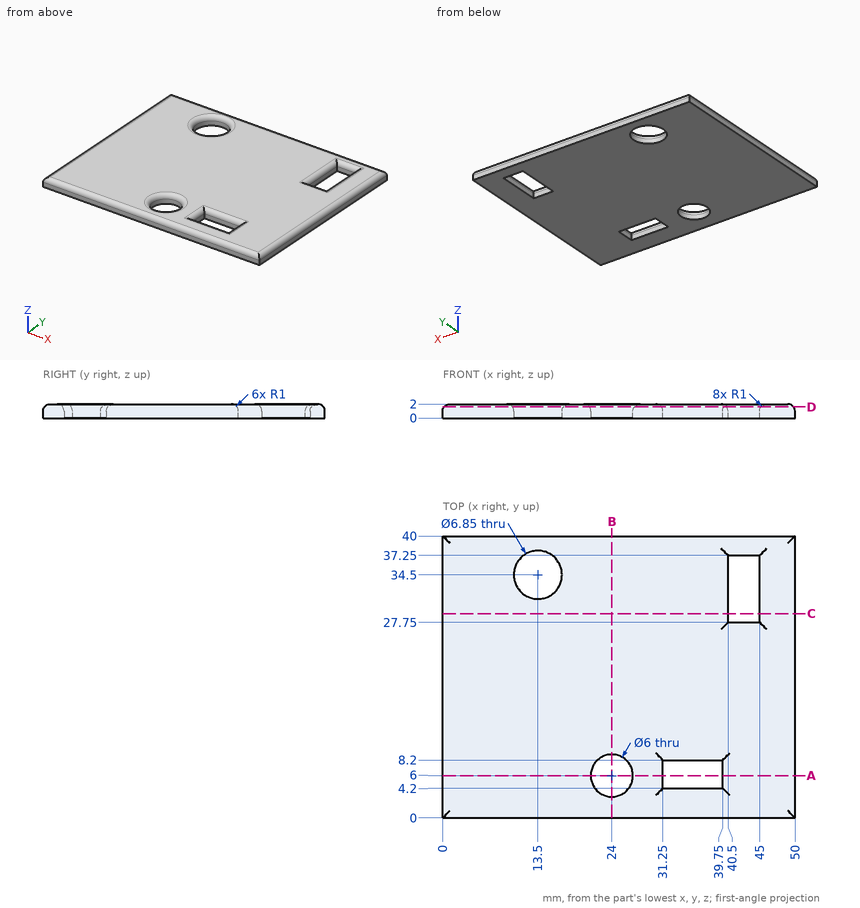
Part print with two shaded views. Sizes in mm from the minimum x, y, z corner. Coordinates: 2 decimals unless noted, no trailing zeros. Order: outer loops, then holes, each group sorted by start corner. A loop starts at its lowest first (then second) coordinate and runs counter-clockwise, first axis right, second up. Notation, with made-up numbers: M 6,46.5 L 18,46.5 A28 ccw 18,67.5 Z; hole C -9.5,83 d3. An arc over 180 degrees is marked long. Use a Markdown table: item, result.
(1) Cut at A-A on y = 6. Write the cut outline in (x, z), then the cut area to 3 significant figures.
A:
| item | result |
|---|---|
| outline | M 0,0 L 21,0 L 21,1 A1 ccw 20,2 L 1,2 A1 ccw 0,1 Z; M 27,0 L 31.25,0 L 31.25,1 A1 ccw 30.25,2 L 28,2 A1 ccw 27,1 Z; M 39.75,0 L 50,0 L 50,1 A1 ccw 49,2 L 40.75,2 A1 ccw 39.75,1 Z |
| area | 69.7 mm^2 |
(2) Probe L1, parallel to Y at x = 13.5, z = 0.3 (3 decimals); L2, parallel to Y at x = 24, z = 0.6; L3, parallel to X at y = 27.5, z = 1.8. List the from-to ranges inside material, lowest first.
A:
| item | result |
|---|---|
| L1 | y = 0 to 31.075, 37.925 to 40 |
| L2 | y = 0 to 3, 9 to 40 |
| L3 | x = 0.4 to 40.1, 45.4 to 49.6 |
(3) Cut at B-B on x = 24. Write the cut outline in (y, z).
A:
| item | result |
|---|---|
| outline | M 0,0 L 3,0 L 3,1 A1 ccw 2,2 L 1,2 A1 ccw 0,1 Z; M 9,0 L 40,0 L 40,1 A1 ccw 39,2 L 10,2 A1 ccw 9,1 Z |
(4) Cut at C-C on y = 29. Write the cut outline in (x, z), then the cut area to 3 significant figures.
A:
| item | result |
|---|---|
| outline | M 0,0 L 40.5,0 L 40.5,1 A1 ccw 39.5,2 L 1,2 A1 ccw 0,1 Z; M 45,0 L 50,0 L 50,1 A1 ccw 49,2 L 46,2 A1 ccw 45,1 Z |
| area | 90.1 mm^2 |
(5) Cut at D-D on z = 1.6. Write the cut outline in (x, y) (3 decimals).
A:
| item | result |
|---|---|
| outline | M 0.2,0.2 L 49.8,0.2 L 49.8,39.8 L 0.2,39.8 Z; hole C 13.5,34.5 d7.25; hole C 24,6 d6.4; hole M 31.05,4 L 39.95,4 L 39.95,8.4 L 31.05,8.4 Z; hole M 40.3,27.55 L 45.2,27.55 L 45.2,37.45 L 40.3,37.45 Z |
(6) Flat gauge pins, fed straight in: pin 1 (0.5 mm diameter, centred on y = 33, z = 0.5, fed in from -X); pin 2 (2 mm diameter, centred on x = 36.5, y = 4.5, fed in from +Z). Where does each tip first touch, or does it go through?
A:
| item | result |
|---|---|
| pin 1 | stops at x = 0 |
| pin 2 | stops at z = 1.95 |
